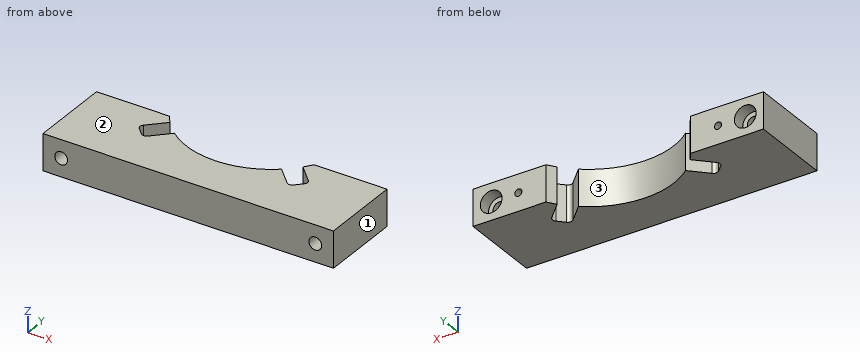
Autodesk Inventor part; units mm, degrees
ref_plane "YZ Plane" through (0, 0, 0) normal (1, 0, 0) x (0, 1, 0)
ref_plane "XZ Plane" through (0, 0, 0) normal (0, 1, 0) x (-1, 0, 0)
ref_plane "XY Plane" through (0, 0, 0) normal (0, 0, 1) x (1, 0, 0)
sketch "Sketch1" plane through (0, 0, 0) normal (0, 0, 1) x (1, 0, 0)
  arc A0 (-50.5454, 57.15) -> (50.5454, 57.15) centre (0, 88.9) ccw
  line L0 (-50.5454, 57.15) -> (-101.6, 57.15)
  line L1 (-101.6, 57.15) -> (-101.6, 0)
  line L2 (-101.6, 0) -> (101.6, 0)
  line L3 (101.6, 0) -> (101.6, 57.15)
  line L4 (101.6, 57.15) -> (50.5454, 57.15)
  line L5 (-142.24, 0) -> (142.24, 0)
  line L6 (0, 57.6383) -> (0, -27.9062) construction
  line L7 (0, -51.2675) -> (0, 112.2612)
  point P0 (0, 0)
  dimension "d32" = 57.15
  dimension "d33" = 59.69
  dimension "d63" = 88.9
  dimension "d64" = 203.2
  dimension "d65" = 101.6
extrude "Extrusion1" add sketch "Sketch1" along normal mid plane 25.4
sketch "Sketch2" plane through (-101.6, 57.15, 12.7) normal (0, 1, 0) x (1, 0, 0)
  line L0 (51.0546, 25.4) -> (51.0546, 0)
  line L1 (51.0546, 0) -> (0, 0)
  line L2 (152.1454, 25.4) -> (152.1454, 0)
  line L3 (203.2, 0) -> (152.1454, 0)
  line L4 (203.2, 25.4) -> (203.2, 0)
  line L5 (0, 0) -> (0, 25.4)
  point P0 (101.6, 12.7)
  point P1 (31.75, 12.7)
  point P2 (171.45, 12.7)
  dimension "d16" = 12.7
  dimension "d18" = 12.7
  dimension "d19" = 31.75
  dimension "d20" = 31.75
hole "Hole1" at (-69.85, 57.15, 0) at (69.85, 57.15, 0) direction (0, -1, 0) diameter 4.9784 depth 25.4
sketch "Sketch4" plane through (0, 0, 12.7) normal (0, 0, 1) x (1, 0, 0)
  line L0 (-46.4578, 51.4224) -> (-59.9282, 37.9521)
  line L1 (-59.9282, 37.9521) -> (-50.9479, 28.9718)
  line L2 (-50.9479, 28.9718) -> (-37.4776, 42.4422)
  line L3 (-37.4776, 42.4422) -> (-46.4578, 51.4224)
  line L4 (37.4776, 42.4422) -> (50.9479, 28.9718)
  line L5 (50.9479, 28.9718) -> (59.9282, 37.9521)
  line L6 (59.9282, 37.9521) -> (46.4578, 51.4224)
  line L7 (46.4578, 51.4224) -> (37.4776, 42.4422)
  line L8 (0, 53.9269) -> (0, 0) construction
  line L9 (-101.6, 0) -> (101.6, 0)
  arc A0 (-50.5454, 57.15) -> (50.5454, 57.15) centre (0, 88.9) ccw
  line L10 (34.6064, 54.2936) -> (52.2131, 36.6869) construction
  line L11 (-58.7882, 30.1118) -> (-24.955, 63.945) construction
  point P0 (46.4578, 51.4224)
  point P1 (-46.4578, 51.4224)
  dimension "d35" = 90
  dimension "d36" = 45
  dimension "d38" = 12.7
  dimension "d39" = 12.7
  dimension "d42" = 6.35
  dimension "d43" = 6.35
  dimension "d46" = 19.05
  dimension "d51" = 19.05
extrude "Extrusion2" cut sketch "Sketch4" against normal through all contours A0 L2 L1 L0 | A0 L6 L5 L4
sketch "Sketch3" plane through (50.5454, 57.15, 12.7) normal (0, 1, 0) x (1, 0, 0)
  line L0 (51.0546, 25.4) -> (51.0546, 0)
  line L1 (51.0546, 0) -> (0, 0)
  line L2 (-152.1454, 0) -> (-152.1454, 25.4)
  line L3 (-101.0907, 0) -> (-152.1454, 0)
  line L4 (-152.1454, 12.7) -> (51.0546, 12.7) construction
  point P0 (-50.5454, 12.7)
  point P1 (38.3546, 12.7)
  point P2 (-139.4454, 12.7)
  dimension "d28" = 12.7
  dimension "d30" = 12.7
hole "Hole2" at (88.9, 57.15, 0) at (-88.9, 57.15, 0) direction (0, -1, 0) diameter 8.89 end through all counterbore diameter 15.24 counterbore depth 8.89
fillet "Fillet2" radius 3.175 4 edges at (-59.9282, 37.9521, 0) (-50.9479, 28.9718, 0) (50.9479, 28.9718, 0) (59.9282, 37.9521, 0)
equation "\"d36\" = 0.5 * d35"
equation "\"d42\" = 0.5 * d39"
equation "\"d43\" = 0.5 * d38"
properties part number "ODSY-0007-003" material "Aluminum 6061"
Geometry: final body of the model. Coordinates: model frame, mm. Face numbers are marked on the shaded views. Give positions to 0.01 mm unless a question says otherwise; leave off trailing zeros. Write each loop counter-clockwise with the first axis right and the second up, starting at its lowest first coordinate (ties: lowest second). Pieces come first, ordered by that corner, then holes. Notation, with made-up numbers: (69.25, 29) - (103.25, 29) arc R19 cw to (103.25, 53) - close; hole circle Ø9 at (-16.5, 20.25). An arc over 180 degrees is marked (long way). Return JSON: item names as keys, results as strings. Group by question number.
1) Section B-B on y = 45.5. Return the cut outline in (x, z) (3 decimals), plus the area to 3 significant figures.
2) Section A-A on x = -88.9. Return the cut outline in (y, z) (3 decimals).
3) Mould query, pull axis X, two halves, no side actions, for the marked faces 1, 2 and 3. Classes: released by +X, released by -X, zero draft, split by the parting line, or undercut.
4) Line query: line 1 (X direction, y = 13, z = 0) (3 decimals); line 2 (Z direction, x = -69.85, y = 46.75); line 3 (X direction, y = 51, z = 0). Output: solid intervals per line, ascending.
5) Section C-C on y = 16.5. Return the cut outline in (x, z) (3 decimals), plus the area to 3 significant figures.
6) Section D-D on z = 0. State how many separate pieces and enclosed holes the cut face has, plus the area to 3 significant figures.
7) First-contact query: P1, Ø4.5, axis at x = -86.5, z = 0, coming from the +Y side; P2, Ø4, axis at x = -69.85, z = 0, coming from the +Y side. Flat tips, straight axial feed; report the tip coordinate or a pass-through.
Filled in:
{
 "1": {"outline": "(-101.6, -12.7) - (-52.38, -12.7) - (-52.38, 12.7) - (-101.6, 12.7) - close; (52.38, -12.7) - (101.6, -12.7) - (101.6, 12.7) - (52.38, 12.7) - close; hole circle Ø8.89 at (-88.9, 0); hole circle Ø4.978 at (-69.85, 0); hole circle Ø4.978 at (69.85, 0); hole circle Ø8.89 at (88.9, 0)", "area": "2,340 mm^2"},
 "2": {"outline": "(0, -12.7) - (57.15, -12.7) - (57.15, -7.62) - (48.26, -7.62) - (48.26, -4.445) - (0, -4.445) - close; (0, 4.445) - (48.26, 4.445) - (48.26, 7.62) - (57.15, 7.62) - (57.15, 12.7) - (0, 12.7) - close"},
 "3": {"face 1": "released by +X", "face 2": "zero draft", "face 3": "undercut"},
 "4": {"line 1": "x = -101.6 to -93.345, -84.455 to 84.455, 93.345 to 101.6", "line 2": "z = -12.7 to -2.49, 2.49 to 12.7", "line 3": "x = -101.6 to -96.52, -81.28 to -72.34, -67.36 to -46.88, 46.88 to 67.36, 72.34 to 81.28, 96.52 to 101.6"},
 "5": {"outline": "(-101.6, -12.7) - (101.6, -12.7) - (101.6, 12.7) - (-101.6, 12.7) - close; hole circle Ø8.89 at (-88.9, 0); hole circle Ø8.89 at (88.9, 0)", "area": "5,040 mm^2"},
 "6": {"separate pieces": "3", "enclosed holes": "0", "area": "7,770 mm^2"},
 "7": {"P1": "stops at y = 48.26", "P2": "stops at y = 31.75"}
}
